Input: part model. Units: mm. Frame: model coordinates. Face numbers are marked on the shaded views. A direction names the side the tool comes from. Coordinates: 2 decimals unless noted, no trailing zeros. Order: outer loops, then holes, each group sorted by start corner. A loop starts at its lowest first (then second) coordinate and runs counter-clockwise, first axis right, second up. Notation, with made-up numbers: M -36.5,44 L -18.5,44 A17 cw -18.5,76 Z; hole C 31,25 d5. An arc over 180 degrees is marked long. One line per item, written item: value.
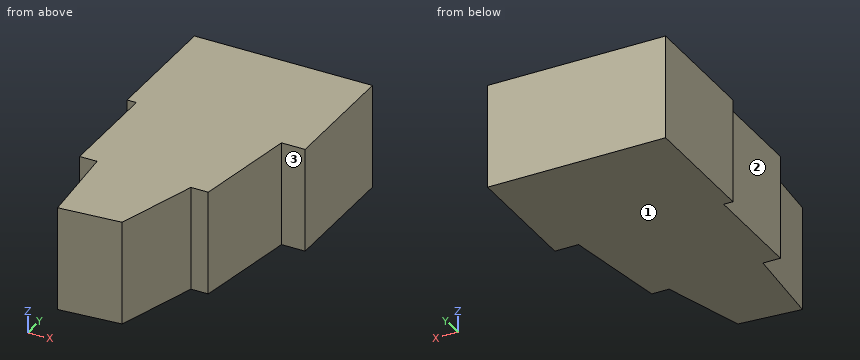
```python
from build123d import *

# Parameters (mm, degrees)
F1_DEPTH = 30.48


with BuildPart() as f1:
    # F0 (on Top) → F1 (new body)
    with BuildSketch(Plane.XY):
        Polygon((-32.288667, -15.490659), (-59.70671, -15.490659), (-57.601184, -40.756974), (-39.528311, -39.250901), align=None)
        Polygon((-22.408817, 15.189869), (-64.820133, 15.189869), (-64.820133, -15.490659), (-59.70671, -15.490659), (-32.288667, -15.490659), (-27.221447, -15.490659), align=None)
        Polygon((-67.527235, 51.585395), (-67.527235, 15.189869), (-64.820133, 15.189869), (-22.408817, 15.189869), (-15.490659, 15.189869), (-15.490659, 51.585395), align=None)
    extrude(amount=F1_DEPTH)


solid = f1.part
```
(1) Cut plane A-A on z = 20.5. Output: boundary loops of the cut face in (x, y).
Data:
outline: M -67.53,15.19 L -64.82,15.19 L -64.82,-15.49 L -59.71,-15.49 L -57.6,-40.76 L -39.53,-39.25 L -32.29,-15.49 L -27.22,-15.49 L -22.41,15.19 L -15.49,15.19 L -15.49,51.59 L -67.53,51.59 Z
(2) Cut plane C-C on y = -32. Output: boundary loops of the cut face in (x, z), plus the area to 3 significant figures.
Data:
outline: M -58.33,0 L -37.32,0 L -37.32,30.48 L -58.33,30.48 Z
area: 640 mm2
(3) Cut plane B-B on x = -26. Output: boundary loops of the cut face in (y, z).
Data:
outline: M -7.7,0 L 51.59,0 L 51.59,30.48 L -7.7,30.48 Z
(4) Access query for the marked faces 1, 2 and 3. Directions: +Z, -Z, +X, -X, +Y, -Y. A direction counts if a zero-diameter tool reaches every point of the face in a straight line with its end or side. Return the directions, or none.
Data:
face 1: -Z, +X, -X, +Y, -Y
face 2: +Z, -Z, -X, -Y
face 3: +Z, -Z, +X, -Y
(5) Ray query, line 1 (Y direction, x = -61.5, z = 22); line 2 (Y direction, x = -19, z = 19.5); line 3 (X direction, y = -35.5, z = 1.5). Return the intervals inside material, ascending. Write a range as from..to.
Data:
line 1: y = -15.49..51.59
line 2: y = 15.19..51.59
line 3: x = -58.04..-38.39
(6) First-contact query: pin 1 (4 mm diameter, centred on x = -63.5, z = 16.5, fed in from -Y); pin 2 (12 mm diameter, centred on y = -4, z = 5, fed in from -X); pin 3 (6 mm diameter, centred on y = 4, z = 7, fed in from +X). Flat tips, straight axial feed; report the tip coordinate or a pass-through.
Data:
pin 1: stops at y = -15.49
pin 2: stops at x = -64.82
pin 3: stops at x = -23.69
